Autodesk Inventor part; units mm, degrees
ref_plane "YZ Plane" through (0, 0, 0) normal (1, 0, 0) x (0, 1, 0)
ref_plane "XZ Plane" through (0, 0, 0) normal (0, 1, 0) x (-1, 0, 0)
ref_plane "XY Plane" through (0, 0, 0) normal (0, 0, 1) x (1, 0, 0)
ref_plane "Arbeitsebene1" through (15, 0, 0) normal (-1, 0, 0) x (0, 1, 0)
sketch "Skizze1" plane through (15, 0, 0) normal (-1, 0, 0) x (0, 1, 0)
  line L0 (32.6031, 0.5) -> (30.7237, 0.5)
  line L1 (30.7237, 4.25) -> (32.6031, 4.25)
  line L2 (30.7237, 0.5) -> (30.7237, 4.25)
  line L3 (32.6031, 0.5) -> (30.7237, 0.5)
  line L4 (30.7237, 4.7) -> (32.6031, 4.7)
  line L5 (30.7237, 0.5) -> (30.7237, 4.25)
  line L6 (30, 0.5) -> (32, 0.5)
  line L7 (30, 0.55) -> (30, 0.5)
  line L8 (32, 0.5) -> (32, 0.55)
  line L9 (32, 0.5) -> (32, 16.1)
  line L10 (52, 0.5) -> (52, 16.1)
  line L11 (42, 19.32) -> (42, -3.22)
  line L12 (32.6031, 0.5) -> (27, 0.5)
  line L13 (27, 0.5) -> (27, -6.5)
  line L14 (27, -6.5) -> (35.6031, -6.5)
  line L15 (35.6031, -6.5) -> (35.6031, 5.25)
  line L16 (35.6031, 5.25) -> (34.1031, 5.25)
  line L17 (32.6031, 0.5) -> (32.6031, 0.2)
  line L18 (32.6031, 0.2) -> (27, 0.2)
  line L19 (32, 0.55) -> (30, 0.55)
  line L20 (32.1031, 0.5) -> (32.0412, 0.2)
  line L21 (27, -6.5) -> (32, -6.5)
  line L22 (32, -6.5) -> (32, -14.5)
  line L23 (32, -14.5) -> (27, -14.5)
  line L24 (27, -14.5) -> (27, -6.5)
  line L25 (34.1031, 5.25) -> (32.307, 3.9176)
  line L26 (32.307, 3.9176) -> (32.1031, 0.5)
  point P0 (0, 0)
  point P1 (30.7237, 0.55)
  point P2 (32, 4.25)
  dimension "d1" = 7
  dimension "d3" = 1
  dimension "d11" = 0.5
  dimension "d13" = 15
  dimension "d14" = 8
  dimension "d15" = 10
  dimension "d37" = 0.3
  dimension "d38" = 6.3969
revolve "Umdrehung1" add sketch "Skizze1" angle 360 about axis through (15, 42, -19.32) along (0, 0, 1) contours L17 L18 L20 L0 | L0 L26 L25 L16 L15 L14 L13 L18 L17
sketch "Skizze2" plane through (0, 0, 0) normal (0, 1, 0) x (-1, 0, 0)
  spline S0 degree 3 poles (-15, -4.25) (-12.1304, -4.4784) (-9.2732, -4.7067) (-7.1109, -4.9351) (-6.8554, -4.962) (-6.6095, -4.989) (-6.3738, -5.016) knots 0 0 0 0 0.7174 0.7174 0.7174 0.802142 0.802142 0.802142 0.802142
  spline S1 degree 3 poles (-14.5016, -1.0897) (-11.6314, -1.3183) (-8.8183, -1.5469) (-6.7355, -1.7755) (-6.2054, -1.8336) (-5.7215, -1.8918) (-5.2918, -1.95) knots 0.041547 0.041547 0.041547 0.041547 0.759706 0.759706 0.759706 0.942478 0.942478 0.942478 0.942478
  circle A0 centre (-15, -2.8138) radius 1.4
  line L0 (-15, 1.0048) -> (-15, -6.0288)
  point P0 (0, 0)
  dimension "d5" = 2.8
extrude "Extrusion1" cut sketch "Skizze2" along normal up to surface
pattern_circular "Runde Anordnung1" count 3 over 360 about axis through (15, 42, 3.15) along (0, 0, -1) of "Extrusion1"
chamfer "Fase1" distance 1 angle 45 1 edges at (15, 48.3969, 6.5)
sketch "Skizze6" plane through (15, 42, 6.5) normal (0, 0, 1) x (1, 0, 0)
  circle A0 centre (0, 0) radius 15
  circle A1 centre (0, 0) radius 7.3969
  circle A2 centre (0, 0) radius 13.15
  circle A3 centre (0, 0) radius 9.5
  point P0 (-15, -42)
  dimension "d31" = 26.3
  dimension "d39" = 19
extrude "Extrusion4" cut sketch "Skizze6" against normal blind 4 contours A1 | A2 | A3
properties part number "30_Linear_Stage_NEMA11_baseholder_bayonetmount_objective_rms_metaladapter_tall"
For this review, take the finished solid that the model builds, in its own axes (mm). A direction names the side the tool comes from. Coordinates: 2 decimals unless noted, no trailing zeros. Write each loop counter-clockwise with the first axis right and the second up, starting at its lowest first coordinate (ties: lowest second). Pieces come first, ordered by that corner, then holes. Notation, with made-up numbers: (-40, 64.25) -> (-6, 64.25) arc R18 ccw to (-6, 70.25) -> close; hole circle Ø4 at (-25.75, 47). An arc over 180 degrees is marked (long way). Write each question's results on one line, items separated by ' | '. Start each with the question number.
1) Consider section C-C (z = 0.75). Write out the cut boundary in (x, y), plus the area to 3 significant figures.
2) Consider section A-A (y = 42). Write out the cut boundary in (x, z).
3) For faces 1 (the face through (12, 32, -0.2)), 2 (the face through (15.303, 33.933, -1.447)), 3 (the face through (12.149, 29.163, 4.528)), list the 3-axis set-ups (+Z, -Z, +X, -X, +Y, -Y) from which the entire face can be reached by the end or side of a thin tool; tool diameter is ignored.
4) The part is to be moulded in two halves that separate along X. For faces 4 (the face through (15.66, 56.985, 3.197)), 5 (the face through (1.7, 42.1, 6.5)), 6 (the face through (14.72, 48.39, -1.43)), say which applies: +X half, -X half, draft (parallel to the pull), parting line (faces both ways), or undercut.
5) Wall thickness on L1, parallel to Z at x = 15, y = 34.45; L2, parallel to X at y = 42, z = -0.5; L3, parallel to Z at x = 10, y = 55: over which ranges is each line inside the solid? List them lowest first. Write a range as [from, to].
6) Consider section D-D (x = 26). Write out the cut boundary in (y, z).
7) Insertion check: pin 1 (3 mm diameter, centred on x = 4, y = 40, fed in from +Z); pin 2 (3 mm diameter, centred on x = 12.5, y = 46, fed in from +Z); pin 3 (3 mm diameter, centred on x = 4.5, y = 33.5, fed in from -Z); pin 4 (2 mm diameter, centred on x = 3.5, z = -0.5, fed in from +Y). Each pin has a flat end and moves straight along its axis. Give the tip position at first contact, or say it passes through.
8) Consider section B-B (x = 15). Write out the cut boundary in (y, z).
Geometry says:
1) outline: circle Ø30 at (15, 42); hole circle Ø12.79 at (15, 42) | area: 578 mm^2
2) outline: (0, -0.2) -> (5.04, -0.2) -> (5.1, -0.5) -> (5.31, -3.92) -> (7.1, -5.25) -> (8.6, -5.25) -> (8.6, 2.5) -> (1.85, 2.5) -> (1.85, 6.5) -> (0, 6.5) -> close; (21.4, -5.25) -> (22.9, -5.25) -> (24.69, -3.92) -> (24.9, -0.5) -> (24.96, -0.2) -> (30, -0.2) -> (30, 6.5) -> (28.15, 6.5) -> (28.15, 2.5) -> (21.4, 2.5) -> close
3) face 1: -Z | face 2: -Y | face 3: +Z
4) face 4: parting line | face 5: draft | face 6: undercut
5) L1: [-5.25, -4.21], [-1.41, 2.5] | L2: [5.1, 8.6], [21.4, 24.9] | L3: [-0.2, 6.5]
6) outline: (31.8, -0.2) -> (52.2, -0.2) -> (52.2, 6.5) -> (49.21, 6.5) -> (49.21, 2.5) -> (34.79, 2.5) -> (34.79, 6.5) -> (31.8, 6.5) -> close
7) pin 1: z = 2.5 | pin 2: through | pin 3: z = -0.2 | pin 4: y = 52.67
8) outline: (27, -0.2) -> (32.04, -0.2) -> (32.1, -0.5) -> (32.16, -1.41) -> (35.6, -1.41) -> (35.6, 2.5) -> (28.85, 2.5) -> (28.85, 6.5) -> (27, 6.5) -> close; (32.71, -4.21) -> (34.1, -5.25) -> (35.6, -5.25) -> (35.6, -4.21) -> close; (48.4, -5.25) -> (49.9, -5.25) -> (51.69, -3.92) -> (51.9, -0.5) -> (51.96, -0.2) -> (57, -0.2) -> (57, 6.5) -> (55.15, 6.5) -> (55.15, 2.5) -> (48.4, 2.5) -> close
